Input: part model. Units: mm. Frame: model coordinates. Face numbers are marked on the shaded views. A direction names the side the tool comes from. Give positions to 0.01 mm unless a question says otherwise; leave off trailing zeros. Write each loop counter-clockwise with the first axis right and the second up, starting at its lowest first coordinate (ties: lowest second). Pieces come first, ordered by that corner, then holes. Notation, with made-up numbers: (23, 31.25) - (57, 31.25) arc R21 ccw to (57, 50.25) - close; hole circle Ø1 at (-19, -19). An arc over 180 degrees is marked (long way). Answer as CSV lines item,"result". Start each with the question number.
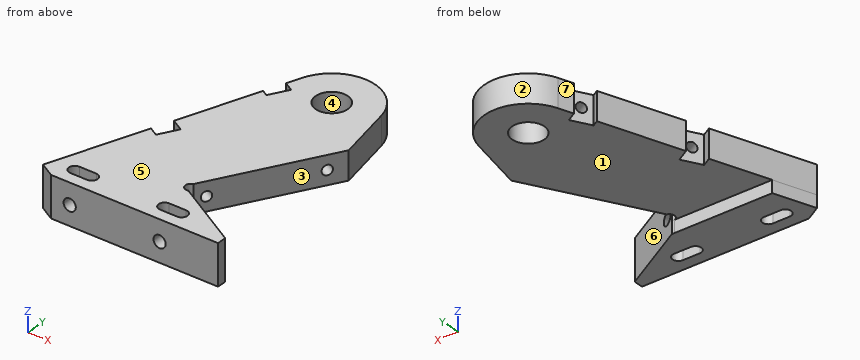
from build123d import *

# Parameters (mm, degrees)
MODEL_R                   = 3.175
BOSS_EXTRUDE1_DEPTH       = 8.4836
F_4_CLEARANCE_HOLE3_D     = 2.9464
F_4_CLEARANCE_HOLE4_D     = 2.9464
BOSS_EXTRUDE2_START       = 3.7084
BOSS_EXTRUDE2_DEPTH       = 3.7084
CUT_EXTRUDE1_DEPTH        = 60.573404892
F_6_CLEARANCE_HOLE2_D     = 3.6576
F_6_CLEARANCE_HOLE2_DEPTH = 14.3256
F_6_CLEARANCE_HOLE2_TIP   = 1.0988539
SKETCH20_R                = 4.826
CUT_EXTRUDE2_DEPTH        = 60.573404892


with BuildPart() as part:
    # Model → Boss-Extrude1 (new body)
    with BuildSketch(Plane.XY):
        with BuildLine():
            Line((30.032015577, -29.521189504), (30.032015577, -26.729824585))
            Line((30.032015577, -26.729824585), (10.04882977, -15.19252688))
            ThreePointArc((10.04882977, -15.19252688), (8.104547287, -14.069994865), (9.227079302, -12.125712382))
            Line((9.227079302, -12.125712382), (29.151876156, 22.3850481))
            Line((29.151876156, 22.3850481), (25.790540116, 39.397524407))
            ThreePointArc((25.790540116, 39.397524407), (13.922877184, 49.944916766), (0.570865514, 41.353485372))
            Line((0.570865514, 41.353485372), (-0.979565285, 37.104375313))
            Line((-0.979565285, 37.104375313), (1.753621818, 35.526369004))
            Line((1.753621818, 35.526369004), (-1.421378182, 30.02710769))
            Line((-1.421378182, 30.02710769), (-3.189468587, 31.047915161))
            Line((-3.189468587, 31.047915161), (-11.768069595, 7.537404491))
            Line((-11.768069595, 7.537404491), (-8.165923931, 5.457704722))
            Line((-8.165923931, 5.457704722), (-11.34077003, -0.041645446))
            Line((-11.34077003, -0.041645446), (-13.977972897, 1.480944339))
            Line((-13.977972897, 1.480944339), (-24.373743148, -27.00969967))
            Line((-24.373743148, -27.00969967), (-20.022585807, -29.521189504))
            Line((-20.022585807, -29.521189504), (30.032015577, -29.521189504))
        make_face()
        with Locations(Location((12.90743615, 36.852072417, 0), (0, 0, 180))):
            Circle(MODEL_R, mode=Mode.SUBTRACT)
    extrude(amount=BOSS_EXTRUDE1_DEPTH)

    # #4 Clearance Hole3 (through all)
    with Locations(Plane(origin=(-14.068152667, 8.12225173, 0), x_dir=(0, 0, 1), z_dir=(-0.8660254037844389, 0.4999999999999996, 0))):
        with Locations((4.2418, 28.46854897)):
            Hole(F_4_CLEARANCE_HOLE3_D / 2)

    # #4 Clearance Hole4 (through all)
    with Locations(Plane(origin=(-8.487819953, 4.900128422, 0), x_dir=(0, 0, 1), z_dir=(-0.8660393963332388, 0.49997576341134725, 0))):
        with Locations((4.2418, -2.53117675)):
            Hole(F_4_CLEARANCE_HOLE4_D / 2)

    # Sketch12 → Boss-Extrude2 (add)
    with BuildSketch(Plane(origin=(0, 0, 0), x_dir=(-1, 0, 0), z_dir=(0, 0, -1)).offset(BOSS_EXTRUDE2_START)):
        with BuildLine():
            Line((20.062967478, -15.195589504), (-9.238684477, -15.195589504))
            ThreePointArc((-9.238684477, -15.195589504), (-9.643955781, -15.246608288), (-10.04882977, -15.19252688))
            Line((-10.04882977, -15.19252688), (-30.032015577, -26.729824585))
            Line((-30.032015577, -26.729824585), (-30.032015577, -29.521189504))
            Line((-30.032015577, -29.521189504), (20.022585807, -29.521189504))
            Line((20.022585807, -29.521189504), (24.373743148, -27.00969967))
            Line((24.373743148, -27.00969967), (20.062967478, -15.195589504))
        make_face()
    extrude(amount=-BOSS_EXTRUDE2_DEPTH)

    # Sketch14 → Cut-Extrude1 (cut, through all)
    with BuildSketch(Plane.XY.offset(8.4836)):
        with BuildLine():
            Line((-16.974585807, -22.485389504), (-11.894585807, -22.485389504))
            ThreePointArc((-11.894585807, -22.485389504), (-10.116585807, -24.263389504), (-11.894585807, -26.041389504))
            Line((-11.894585807, -26.041389504), (-16.974585807, -26.041389504))
            ThreePointArc((-16.974585807, -26.041389504), (-18.752585807, -24.263389504), (-16.974585807, -22.485389504))
        make_face()
        with BuildLine():
            Line((9.966182511, -22.485389504), (15.046182511, -22.485389504))
            ThreePointArc((15.046182511, -22.485389504), (16.824182511, -24.263389504), (15.046182511, -26.041389504))
            Line((15.046182511, -26.041389504), (9.966182511, -26.041389504))
            ThreePointArc((9.966182511, -26.041389504), (8.188182511, -24.263389504), (9.966182511, -22.485389504))
        make_face()
    extrude(amount=-CUT_EXTRUDE1_DEPTH, mode=Mode.SUBTRACT)

    # #6 Clearance Hole2
    with Locations(Plane(origin=(0, -29.521189504, 0), x_dir=(-1, 0, 0), z_dir=(0, -1, 0))):
        with Locations((14.433829056, -2.212184194), (-12.506939307, -2.212184194)):
            Hole(F_6_CLEARANCE_HOLE2_D / 2, depth=F_6_CLEARANCE_HOLE2_DEPTH)
            with Locations((0, 0, -(F_6_CLEARANCE_HOLE2_DEPTH + F_6_CLEARANCE_HOLE2_TIP / 2))):  # 118° drill point
                Cone(0, F_6_CLEARANCE_HOLE2_D / 2, F_6_CLEARANCE_HOLE2_TIP, mode=Mode.SUBTRACT)

    # Sketch20 → Cut-Extrude2 (cut, through all)
    with BuildSketch(Plane.XY.offset(8.4836)):
        with Locations((12.90743615, 36.852072417)):
            Circle(SKETCH20_R)
    extrude(amount=-CUT_EXTRUDE2_DEPTH, mode=Mode.SUBTRACT)


solid = part.part
1) Pull-direction query (Y, two-part tool) for the marked faces 4, 5, 6 and 7; classes: +Y half, -Y half, draft (parallel to the pull), parting line (faces both ways), or undercut.
2) Cut plane B-B on y = 38. Output: boundary loops of the cut face in (x, z).
3) Cut plane D-D on z = 6.5. Output: boundary loops of the cut face in (x, y) (1 decimal).
4) Contact query for flat-ended pins moving along their axis: P1, Ø12, axis at x = 4.5, y = -6, coming from the -Z side; P2, Ø2, axis at y = 0, z = 6, coming from the +X side; P3, Ø4, axis at x = -15.5, z = -0.5, coming from the +Y side. Output: stop coordinate, or through.
5) Cut plane A-A on z = -1. Output: boundary loops of the cut face in (x, y) (1 decimal), and give its area (3 significant figures).
6) Reachability of the marked faces 1, 2 and 3 from +Z, -Z, +X, -X, +Y, -Y: full face, straight path, thin tool, end or side. Return the list, or none.
7) Cut plane C-C on y = -21. Output: boundary loops of the cut face in (x, z).
8) Material intervals for line 1 (Y direction, x = 10, z = -0.25); line 2 (Y direction, x = 15, z = 7.25); line 3 (Y direction, x = 22, z = 4.5), sorted ascending. Write a range as from..to.
Numbers:
1,face 4,"undercut"
1,face 5,"draft"
1,face 6,"undercut"
1,face 7,"+Y half"
2,outline,"(-0.65, 0) - (8.22, 0) - (8.22, 8.48) - (-0.65, 8.48) - close; (17.59, 0) - (26.07, 0) - (26.07, 8.48) - (17.59, 8.48) - close"
3,outline,"(-24.4, -27) - (-20, -29.5) - (30, -29.5) - (30, -26.7) - (10, -15.2) arc R1.6 cw to (9.2, -12.1) - (29.2, 22.4) - (25.8, 39.4) arc R13.1 ccw to (0.6, 41.4) - (-1, 37.1) - (1.8, 35.5) - (-1.4, 30) - (-3.2, 31) - (-11.8, 7.5) - (-8.2, 5.5) - (-11.3, 0) - (-14, 1.5) - close; hole (-17, -26) - (-11.9, -26) arc R1.8 ccw to (-11.9, -22.5) - (-17, -22.5) arc R1.8 ccw to start; hole circle Ø9.7 at (12.9, 36.9); hole (10, -26) - (15, -26) arc R1.8 ccw to (15, -22.5) - (10, -22.5) arc R1.8 ccw to start"
4,P1,"stops at z = 0"
4,P2,"stops at x = 16.81"
4,P3,"stops at y = 1.48"
5,outline,"(-24.4, -27) - (-20, -29.5) - (30, -29.5) - (30, -26.7) - (10, -15.2) arc R1.6 cw to (9.2, -15.2) - (-20.1, -15.2) - close; hole (-17, -26) - (-11.9, -26) arc R1.8 ccw to (-11.9, -22.5) - (-17, -22.5) arc R1.8 ccw to start; hole (10, -26) - (15, -26) arc R1.8 ccw to (15, -22.5) - (10, -22.5) arc R1.8 ccw to start"
5,area,"577 mm²"
6,face 1,"-Z, +X, -X, +Y"
6,face 2,"+Z, -Z, +Y"
6,face 3,"+Z, -Z, +X"
7,outline,"(-22.18, -3.71) - (20.11, -3.71) - (20.11, 8.48) - (-22.18, 8.48) - close; hole circle Ø3.66 at (-14.43, 2.21); hole circle Ø3.66 at (12.51, 2.21)"
8,line 1,"y = -29.52..-26.04, -22.49..-15.2"
8,line 2,"y = -29.52..-26.04, -22.49..-18.05, -2.13..32.5, 41.2..49.82"
8,line 3,"y = -29.52..-22.09, 10..18.5, 21.85..46.33"
